```python
from build123d import *

# Parameters (mm, degrees)
F0_W     = 101.6
F0_H     = 254
F0_R     = 1.7272
F0_W_2   = 24
F0_H_2   = 12.254687
F1_DEPTH = 6.35
F2_W     = 101.6
F2_H     = 254
F2_W_2   = 88.9
F2_H_2   = 241.3
F3_DEPTH = 76.2
F4_R     = 1.5
F4_R_2   = 11.253
F5_DEPTH = 6.35
F6_DEPTH = 6.35


with BuildPart() as f1:
    # F0 (on Top) → F1 (new body)
    with BuildSketch(Plane.XY):
        with Locations((50.8, -127)):
            Rectangle(F0_W, F0_H)
        with Locations((10.31875, -250.03125)):
            Circle(F0_R, mode=Mode.SUBTRACT)
        with Locations((18.35, -235.387502)):
            Rectangle(F0_W_2, F0_H_2, mode=Mode.SUBTRACT)
        with Locations((10.31875, -220.743755)):
            Circle(F0_R, mode=Mode.SUBTRACT)
        with Locations((83.25, -235.387502)):
            Rectangle(F0_W_2, F0_H_2, mode=Mode.SUBTRACT)
        with Locations((91.28125, -250.03125)):
            Circle(F0_R, mode=Mode.SUBTRACT)
        with Locations((91.28125, -220.743755)):
            Circle(F0_R, mode=Mode.SUBTRACT)
        with Locations((10.31875, -33.256245)):
            Circle(F0_R, mode=Mode.SUBTRACT)
        with Locations((10.31875, -3.96875)):
            Circle(F0_R, mode=Mode.SUBTRACT)
        with Locations((18.35, -18.612497)):
            Rectangle(F0_W_2, F0_H_2, mode=Mode.SUBTRACT)
        with Locations((91.28125, -33.256245)):
            Circle(F0_R, mode=Mode.SUBTRACT)
        with Locations((83.25, -18.612497)):
            Rectangle(F0_W_2, F0_H_2, mode=Mode.SUBTRACT)
        with Locations((91.28125, -3.96875)):
            Circle(F0_R, mode=Mode.SUBTRACT)
    extrude(amount=F1_DEPTH)

    # F2 (on face) → F3 (join)
    with BuildSketch(Plane.XY.offset(6.35)):
        with Locations((50.8, -127)):
            Rectangle(F2_W, F2_H)
        with Locations((50.8, -127)):
            Rectangle(F2_W_2, F2_H_2, mode=Mode.SUBTRACT)
    extrude(amount=F3_DEPTH)

    # F4 (on face) → F5 (cut, through all)
    with BuildSketch(Plane(origin=(0, 0, 0), x_dir=(-1, 0, 0), z_dir=(0, 1, 0))):
        with Locations((-66.299994, 76.547002)):
            Circle(F4_R)
        with Locations((-35.300006, 76.547002)):
            Circle(F4_R)
        with Locations((-66.299994, 45.547013)):
            Circle(F4_R)
        with Locations((-50.8, 61.047008)):
            Circle(F4_R_2)
        with Locations((-35.300006, 45.547013)):
            Circle(F4_R)
    extrude(amount=-F5_DEPTH, mode=Mode.SUBTRACT)

    # F4 (on face) → F6 (cut, through all)
    with BuildSketch(Plane(origin=(0, 0, 0), x_dir=(-1, 0, 0), z_dir=(0, 1, 0))):
        with Locations((-66.299994, 76.547002)):
            Circle(F4_R)
        with Locations((-35.300006, 76.547002)):
            Circle(F4_R)
        with Locations((-66.299994, 45.547013)):
            Circle(F4_R)
        with Locations((-50.8, 61.047008)):
            Circle(F4_R_2)
        with Locations((-35.300006, 45.547013)):
            Circle(F4_R)
    extrude(amount=-F6_DEPTH, mode=Mode.SUBTRACT)


solid = f1.part
```
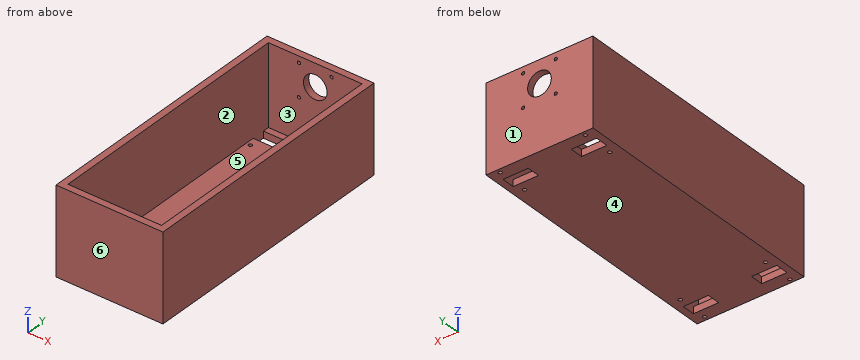
Could you check a few things on this model? Use its own coordinates, in mm. Face numbers are marked on the shaded views. A direction names the side the tool comes from. Round coordinates to 2 decimals unless told otherwise and drop trailing zeros. Write each loop counter-clockwise with the first axis right and the second up, starting at its lowest first coordinate (ties: lowest second). Pieces come first, ordered by that corner, then holes. Notation, with made-up numbers: M 33,86.5 L 86,86.5 A17 cw 86,112.5 Z; hole C 65.5,-4.75 d6. An arc over 180 degrees is marked long. Write each question's results on one line, items separated by ' | '. Start each with the question number.
1. On a 3-axis mill with a long thin cutter (end or side, diameter ignored), from which of +Z, -Z, +X, -X, +Y, -Y can I reach the whole of each face in a straight line? I mean the marked faces 1 and 2. Say none if no direction works.
2. I need wall thicknesses on L1, parallel to X at y = -71, z = 31; L2, parallel to Y at x = 7, z = 29.5. Which ranges of each line are inside material? Lowest first, please. Write a range as from..to.
3. Imagine slicing it at C-C on x = 50.8. List the corners of the cut face in (y, z) for me, and give its area (3 significant figures).
4. Imagine slicing it at B-B on y = -58. List the corners of the cut face in (x, z) for me.
5. I'm going to push flat-ended pins straight in: pin 1 Ø5 at (x, z) = (13, 4) entering from +Y; pin 2 Ø2 at (x, z) = (55, 67) entering from +Y; pin 3 Ø2 at (x, y) = (10.32, -33.26) entering from -Z. Where does each tip first touch, or does it pass through?
6. Thinking about a two-plate mould opening in Y: for the marked faces 3, 4, 5 and 6, which applies, +Y half, -Y half, draft (parallel to the pull), parting line (faces both ways), or undercut?
7. Imagine slicing it at A-A on x = 81.5. List the corners of the cut face in (y, z) for me.
Result sheet:
1) face 1: +Z, -Z, +X, -X, +Y | face 2: +Z
2) L1: x = 0..6.35, 95.25..101.6 | L2: y = -254..-247.65, -6.35..0
3) outline: M -254,0 L 0,0 L 0,49.79 L -6.35,49.79 L -6.35,6.35 L -247.65,6.35 L -247.65,82.55 L -254,82.55 Z; M -6.35,72.3 L 0,72.3 L 0,82.55 L -6.35,82.55 Z | area: 2,440 mm^2
4) outline: M 0,0 L 101.6,0 L 101.6,82.55 L 95.25,82.55 L 95.25,6.35 L 6.35,6.35 L 6.35,82.55 L 0,82.55 Z
5) pin 1: stops at y = 0 | pin 2: stops at y = -247.65 | pin 3: passes through
6) face 3: undercut | face 4: draft | face 5: undercut | face 6: -Y half
7) outline: M -254,0 L -241.51,0 L -241.51,6.35 L -247.65,6.35 L -247.65,82.55 L -254,82.55 Z; M -229.26,0 L -24.74,0 L -24.74,6.35 L -229.26,6.35 Z; M -12.49,0 L 0,0 L 0,82.55 L -6.35,82.55 L -6.35,6.35 L -12.49,6.35 Z
